Part print with two shaded views. Sizes in mm from the minimum x, y, z corner. Give positions to 0.01 mm unless a question says otherwise; leave off trailing zeros. Order: outer loops, then holes, each group sorted by start corner. A loop starts at its lowest first (then second) coordinate and runs counter-clockwise, first axis right, second up. Notation, with made-up numbers: M 53,87 L 95,87 A27 ccw 95,122 Z; hole C 0.25,-6 d8. An arc over 180 degrees is marked long. Return JSON: item names as keys, results as strings.
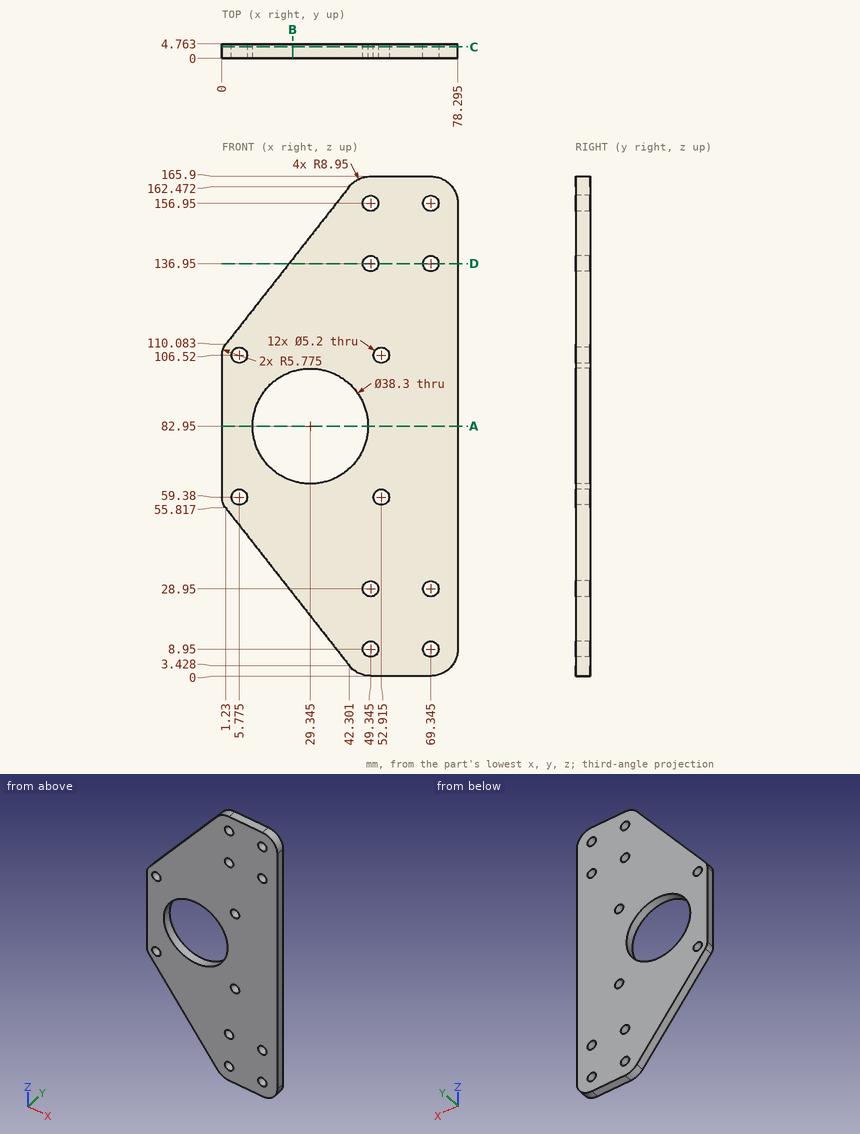
Q1. Band-saw the part on C-C (y = 3.8). Give the number of separate pieces and of enclosed holes in the cut face, then the cut area to 3 significant figures.
Established:
{"separate pieces": "1", "enclosed holes": "13", "area": "8,960 mm²"}
Q2. Band-saw the part on D-D (z = 136.95). Give the cut face in (x, y) (1 decimal), then the cut area to 3 significant figures.
Established:
{"outline": "M 22.3,0 L 46.7,0 L 46.7,4.8 L 22.3,4.8 Z; M 51.9,0 L 66.7,0 L 66.7,4.8 L 51.9,4.8 Z; M 71.9,0 L 78.3,0 L 78.3,4.8 L 71.9,4.8 Z", "area": "217 mm²"}
Q3. Band-saw the part on A-A (z = 82.95). Give the cut face in (x, y) (1 decimal).
Established:
{"outline": "M 0,0 L 10.2,0 L 10.2,4.8 L 0,4.8 Z; M 48.5,0 L 78.3,0 L 78.3,4.8 L 48.5,4.8 Z"}
Q4. Pin check, flat tips, straight feed: pin 1 (8.5 mm diameter, centred on x = 69.345, z = 136.95, fed in from +Y); pin 2 (4.5 mm diameter, centred on x = 49.345, z = 136.95, fed in from +Y); pin 3 (2 mm diameter, centred on y = 2, z = 57, fed in from -X). Stop position of each tip, or through.
Established:
{"pin 1": "stops at y = 4.76", "pin 2": "passes through", "pin 3": "stops at x = 0.17"}
Q5. Probe line 1 along X through (y, z) = (4.3, 137.5) (1 decimal); line 2 along X through (y, z) = (1.1, 108) (1 decimal); line 3 along Z through (x, y) = (69, 1). List the from-to ranges inside material, lowest first.
Established:
{"line 1": "x = 22.7 to 46.8, 51.9 to 66.8, 71.9 to 78.3", "line 2": "x = 0.2 to 3.6, 7.9 to 50.8, 55.1 to 78.3", "line 3": "z = 0 to 6.37, 11.53 to 26.37, 31.53 to 134.37, 139.53 to 154.37, 159.53 to 165.9"}
Q6. Band-saw the part on B-B (x = 23.5). Give the cut face in (y, z), then the cut area to 3 significant figures.
Established:
{"outline": "M 0,27.41 L 4.76,27.41 L 4.76,64.71 L 0,64.71 Z; M 0,101.19 L 4.76,101.19 L 4.76,138.49 L 0,138.49 Z", "area": "355 mm²"}
